Check sheet for the modelled part. Datum: model origin and axes. Units: mm. Face numbers are marked on the shaded views. A direction names the side the tool comes from. Round coordinates to 2 decimals unless told otherwise and drop trailing zeros. Write each loop counter-clockwise with the first axis right and the second up, starting at its lowest first coordinate (ties: lowest second). Pieces come first, ordered by that corner, then holes. Notation, with made-up numbers: (77, 14) - (86, 14) arc R26 cw to (86, 53) - close; hole circle Ø5 at (-37.75, 50). An arc over 180 degrees is marked (long way). Answer as a JSON object with one key per item and string values. Group by question number.
Item 1: Sectioned sample at C-C on z = -3.25. Record the boundary of the cut face in (x, y), plus the area to 3 significant figures.
Item 2: Sectioned sample at B-B on x = 7. Record the boundary of the cut face in (y, z), plus the area to 3 significant figures.
Item 3: Sectioned sample at A-A on y = 0. Record the boundary of the cut face in (x, z).
Item 4: Thickness scan on line 1 (Y direction, x = 10.5, z = -3.5); line 2 (Y direction, x = 5.75, z = -2); line 3 (Z direction, x = 9, y = 1). Record the ranges inside material, lowest first.
Item 5: Set-up check for the marked faces 4 and 5: record each of +Z, -Z, +X, -X, +Y, -Y from which the full face is reachable in a straight line by a thin tool's end or side.
Item 6: Gauge pin test, flat ends, axial feed: P1, Ø4, axis at y = -1, z = -1.5, coming from the +X side; P2, Ø1, axis at x = 8.5, y = 4, coming from the +Z side; P3, Ø1, axis at x = 6, z = 3.5, coming from the -Y side; P4, Ø5, axis at x = 8, z = -4.5, coming from the -Y side. Record the tip position at first contact, or that the pin passes through.
Item 7: Release check for a two-part mould opening along Z. For the marked faces 1, 2 and 3 record: pulls with the +Z half, pulls with the -Z half, needs draft (parallel to the pull), parting line crosses it, or undercut.
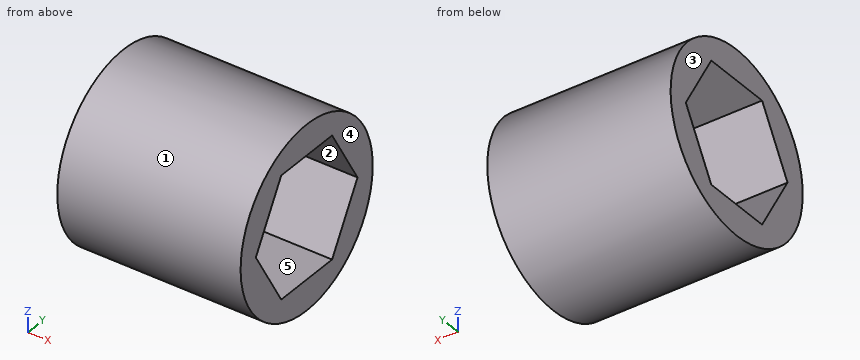
```python
from build123d import *

# Parameters (mm, degrees)
BUSHING_PROFILE_R = 6.35
BUSHING_DEPTH     = 12.7


with BuildPart() as part:
    # Bushing Profile → Bushing (new body)
    with BuildSketch(Plane(origin=(0, 0, 0), x_dir=(0, 0, -1), z_dir=(1, 0, 0))):
        Circle(BUSHING_PROFILE_R)
        Polygon((0, -4.8895), (4.234431212, -2.44475), (4.234431212, 2.44475), (0, 4.8895), (-4.234431212, 2.44475), (-4.234431212, -2.44475), align=None, mode=Mode.SUBTRACT)
    extrude(amount=BUSHING_DEPTH)


solid = part.part
```
Completed:
{
 "1": {"outline": "(0, -5.46) - (12.7, -5.46) - (12.7, -3.01) - (0, -3.01) - close; (0, 3.01) - (12.7, 3.01) - (12.7, 5.46) - (0, 5.46) - close", "area": "62.0 mm²"},
 "2": {"outline": "circle Ø12.7 at (0, 0); hole (-4.89, 0) - (-2.44, -4.23) - (2.44, -4.23) - (4.89, 0) - (2.44, 4.23) - (-2.44, 4.23) - close", "area": "64.6 mm²"},
 "3": {"outline": "(0, -6.35) - (12.7, -6.35) - (12.7, -4.23) - (0, -4.23) - close; (0, 4.23) - (12.7, 4.23) - (12.7, 6.35) - (0, 6.35) - close"},
 "4": {"line 1": "-5.3 to -2.87, 2.87 to 5.3", "line 2": "-6.03 to -3.73, 3.73 to 6.03", "line 3": "-6.27 to -4.23, 4.23 to 6.27"},
 "5": {"face 4": "+Z, -Z, +X, +Y, -Y", "face 5": "+X, -X"},
 "6": {"P1": "through", "P2": "z = 5.3", "P3": "y = -5.6", "P4": "y = -6.03"},
 "7": {"face 1": "parting line crosses it", "face 2": "undercut", "face 3": "needs draft"}
}
